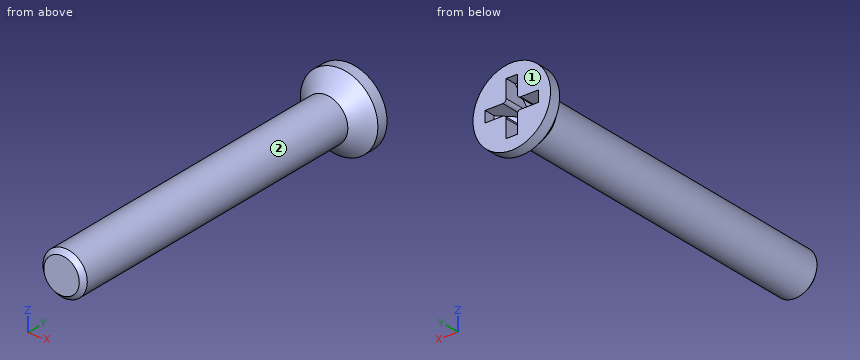
```python
from build123d import *

# Parameters (mm, degrees)
SKETCH_2_W               = 0.5
SKETCH_2_H               = 1.2
CUT_EXTRUDE_1_DEPTH      = 0.5
CUT_EXTRUDE_2_DEPTH      = 0.5
PATTERN_CIRCULAR_1_COUNT = 4
FILLET_1_R               = 0.15


with BuildPart() as part:
    # 草图1 → 旋转1 (revolve)
    with BuildSketch(Plane.XY, mode=Mode.PRIVATE) as revolve_1_sk:
        Polygon((0, 2.689659811), (-1.75, 2.689659811), (-1.75, 2.179659811), (-1, 1.429659811), (-1, -13.110340189), (-0.8, -13.310340189), (0, -13.310340189), align=None)
    revolve(revolve_1_sk.sketch.rotate(Axis((0, -3.769198969, 0), (0, 1, 0)), 270), axis=Axis((0, -3.769198969, 0), (0, 1, 0)))

    # 草图2 → 切除-拉伸1 (cut)
    with BuildSketch(Plane(origin=(0, 2.689659811, 0), x_dir=(1, 0, 0), z_dir=(0, 1, 0))):
        with Locations((0, 0.6)):
            Rectangle(SKETCH_2_W, SKETCH_2_H)
    cut_extrude_1 = extrude(amount=-CUT_EXTRUDE_1_DEPTH, mode=Mode.SUBTRACT)

    # 草图3 → 切除-拉伸2 (cut)
    with BuildSketch(Plane(origin=(-0.25, 0, 0), x_dir=(0, 0, -1), z_dir=(1, 0, 0))):
        Polygon((0, 2.189659811), (0, 1.429659811), (0.44, 1.429659811), (1.2, 2.189659811), align=None)
    cut_extrude_2 = extrude(amount=CUT_EXTRUDE_2_DEPTH, mode=Mode.SUBTRACT)

    # 阵列(圆周)1: 切除-拉伸1, 切除-拉伸2 ×4 about axis
    pattern_circular_1_axis = Axis((0, 0, 0), (0, 1, 0))
    add([cut_extrude_1.rotate(pattern_circular_1_axis, i * 360 / PATTERN_CIRCULAR_1_COUNT) for i in range(1, PATTERN_CIRCULAR_1_COUNT)], mode=Mode.SUBTRACT)
    add([cut_extrude_2.rotate(pattern_circular_1_axis, i * 360 / PATTERN_CIRCULAR_1_COUNT) for i in range(1, PATTERN_CIRCULAR_1_COUNT)], mode=Mode.SUBTRACT)

    # 圆角1
    fillet_1_edges = [part.edges().sort_by_distance(p)[0] for p in [
        (0.25, 2.059659811, -0.25),
        (-0.25, 2.059659811, -0.25),
        (0.25, 2.059659811, 0.25),
        (-0.25, 2.059659811, 0.25),
    ]]
    fillet(fillet_1_edges, radius=FILLET_1_R)


solid = part.part
```
The model under review builds one solid part; all positions refer to its coordinate system, in mm. Face numbers are marked on the shaded views. A direction names the side the tool comes from. Round coordinates to 2 decimals unless told otherwise and drop trailing zeros. Loops run counter-clockwise (first coordinate to the right, second up) from the corner with the lowest first, then second, coordinate; pieces in that order, holes last. Notation, with made-up numbers: (51, -37) - (109, -37) arc R20 ccw to (109, -33) - close; hole circle Ø8 at (78.25, 71). An arc over 180 degrees is marked (long way). Use a Markdown table: item, result. Add a question column.
Q1. Add section A-A (y = 1.75). State the section outline as (x, z) points.
Q2. Insertion check: pin 1 Ø0.6 at (y, z) = (2, -0.5) entering from -X; pin 2 Ø0.6 at (y, z) = (2, -1) entering from +X; pin 3 Ø0.9 at (x, y) = (-1, 2) entering from -Z. Each pin has a flat end and moves straight along its axis. Give the tip position at first contact, or say it passes through.
Q3. Machinability: for the marked faces 1 and 2, which of the approach directions +Z, -Z, +X, -X, +Y, -Y give a long, thin tool a straight path to every point of the face, cutting with its end or side? Answer none if there is none.
Q4. Add section C-C (z = 0). State the section outline as (x, y) points, plus the area to 3 significant figures.
Q5. For probe 1 along X at (y, z) = (-11.5, 0.6); probe 2 along Z at (x, y) = (-0.2, -10), list the stretches that pass through material, from the lowest coordinate up.
Q6. Add section D-D (y = -5). State the section outline as (x, z) points, plus the area to 3 significant figures.
Q7. Add section B-B (x = 0). State the section outline as (y, z) points.
Worked answers:
| question | item | result |
|---|---|---|
| 1 | outline | circle Ø2.64 at (0, 0); hole (-0.76, -0.25) - (-0.4, -0.25) arc R0.15 cw to (-0.25, -0.4) - (-0.25, -0.76) - (0.25, -0.76) - (0.25, -0.4) arc R0.15 cw to (0.4, -0.25) - (0.76, -0.25) - (0.76, 0.25) - (0.4, 0.25) arc R0.15 cw to (0.25, 0.4) - (0.25, 0.76) - (-0.25, 0.76) - (-0.25, 0.4) arc R0.15 cw to (-0.4, 0.25) - (-0.76, 0.25) - close |
| 2 | pin 1 | x = -1.73 |
| 2 | pin 2 | x = 1.58 |
| 2 | pin 3 | z = -1.65 |
| 3 | face 1 | +Z, -Z, +X, -X, +Y |
| 3 | face 2 | -Y |
| 4 | outline | (-1.75, 2.18) - (-1, 1.43) - (-1, -13.11) - (-0.8, -13.31) - (0.8, -13.31) - (1, -13.11) - (1, 1.43) - (1.75, 2.18) - (1.75, 2.69) - (1.2, 2.69) - (1.2, 2.19) - (0.44, 1.43) - (-0.44, 1.43) - (-1.2, 2.19) - (-1.2, 2.69) - (-1.75, 2.69) - close |
| 4 | area | 30.8 mm² |
| 5 | probe 1 | -0.8 to 0.8 |
| 5 | probe 2 | -0.98 to 0.98 |
| 6 | outline | circle Ø2 at (0, 0) |
| 6 | area | 3.14 mm² |
| 7 | outline | (-13.31, -0.8) - (-13.11, -1) - (1.43, -1) - (2.18, -1.75) - (2.69, -1.75) - (2.69, -1.2) - (2.19, -1.2) - (1.43, -0.44) - (1.43, 0.44) - (2.19, 1.2) - (2.69, 1.2) - (2.69, 1.75) - (2.18, 1.75) - (1.43, 1) - (-13.11, 1) - (-13.31, 0.8) - close |
